```python
from build123d import *

# Parameters (mm, degrees)
SKETCH1_R               = 63.5
BOSS_EXTRUDE1_DEPTH     = 762
CUT_EXTRUDE1_DEPTH      = 1032.82015403
CUT_EXTRUDE1_DEPTH_BACK = 387.260908
SKETCH2_W               = 765.404618736
SKETCH2_H               = 508
SKETCH3_R               = 38.1
BOSS_EXTRUDE2_DEPTH     = 203.2
FILLET1_R               = 25.4


with BuildPart() as part:
    # Sketch1 → Boss-Extrude1 (new body)
    with BuildSketch(Plane.XY):
        with BuildLine():
            Line((-475.33654421, 0), (32.66345579, 0))
            Line((32.66345579, 0), (32.66345579, 508))
            ThreePointArc((32.66345579, 508), (-317.204687381, 440.127182905), (-475.33654421, 120.739091765))
            Line((-475.33654421, 120.739091765), (-475.33654421, 0))
        make_face()
        with Locations((-94.33654421, 378.291313639)):
            Circle(SKETCH1_R, mode=Mode.SUBTRACT)
    extrude(amount=BOSS_EXTRUDE1_DEPTH)

    # Sketch2 → Cut-Extrude1 (cut, two sides: drawn at the far end of the back side and taken through both)
    with BuildSketch(Plane(origin=(0, 508, 0), x_dir=(1, 0, 0), z_dir=(0, 1, 0)).offset(-CUT_EXTRUDE1_DEPTH_BACK)):
        with Locations((-173.345287356, -381)):
            Rectangle(SKETCH2_W, SKETCH2_H)
    extrude(amount=CUT_EXTRUDE1_DEPTH + CUT_EXTRUDE1_DEPTH_BACK, mode=Mode.SUBTRACT)

    # Sketch3 → Boss-Extrude2 (add)
    with BuildSketch(Plane.XY.offset(762)):
        with Locations(Location((-333.507660116, 140.616973841, 0), (0, 0, 180))):
            Circle(SKETCH3_R)
    boss_extrude2 = extrude(amount=BOSS_EXTRUDE2_DEPTH)

    # Mirror1: Boss-Extrude2 across plane
    add(boss_extrude2.mirror(Plane.XY.offset(381)))

    # Fillet1
    fillet1_edges = [part.edges().sort_by_distance(p)[0] for p in [
        (32.66345579, 508, 63.5),
        (32.66345579, 508, 698.5),
    ]]
    fillet(fillet1_edges, radius=FILLET1_R)


solid = part.part
```
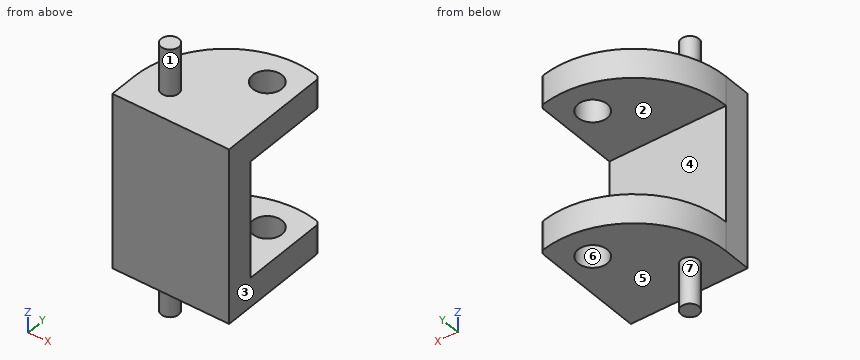
The listing builds one solid part. Answer for the finished solid, in the listing's coordinates (mm). Face numbers are marked on the shaded views. A direction names the side the tool comes from. Coordinates: 2 decimals unless noted, no trailing zeros. Loops run counter-clockwise (first coordinate to the right, second up) from the corner with the lowest first, then second, coordinate; pieces in that order, holes last. Notation, with made-up numbers: (83, -29.75) - (123, -29.75) arc R27 ccw to (123, -11.75) - close; hole circle Ø6 at (86.25, 6). An arc over 180 degrees is marked (long way). Write item = value, one per line.
1) Section B-B (x = -131) is taken. Determine the outline of the cut face in (y, z) (3 decimals).
Responses:
outline = (0, 0) - (326.445, 0) - (326.445, 127) - (120.739, 127) - (120.739, 635) - (326.445, 635) - (326.445, 762) - (0, 762) - close; (430.138, 0) - (518.244, 0) - (518.244, 127) - (430.138, 127) - close; (430.138, 635) - (518.244, 635) - (518.244, 762) - (430.138, 762) - close
2) Which of the six approach directions +Z, -Z, +X, -X, +Y, -Y give full straight-line access (tool end or side, diameter ignored) to the marked faces 1, 2 and 3?
Responses:
face_1 = +Z
face_2 = +X, -X, +Y
face_3 = +Z, -Z, +X, +Y, -Y
3) Section C-C (y = 470) is taken. Determine the outline of the cut face in (x, z).
Responses:
outline = (-271.99, 0) - (32.66, 0) - (32.66, 127) - (-271.99, 127) - close; (-271.99, 635) - (32.66, 635) - (32.66, 762) - (-271.99, 762) - close
4) Determine the mould class of the marked faces 4, 5, 6 and 7 for opening direction Y: pulls with the +Y half, pulls with the -Y half, needs draft (parallel to the pull), parting line crosses it, or undercut.
Responses:
face_4 = pulls with the +Y half
face_5 = needs draft
face_6 = undercut
face_7 = parting line crosses it
5) Section D-D (z = 552.5) is taken. Determine the outline of the cut face in (x, y).
Responses:
outline = (-475.34, 0) - (32.66, 0) - (32.66, 120.74) - (-475.34, 120.74) - close
6) Section A-A (y = 407) is taken. Determine the outline of the cut face in (x, z).
Responses:
outline = (-355.41, 0) - (-150.98, 0) - (-150.98, 127) - (-355.41, 127) - close; (-355.41, 635) - (-150.98, 635) - (-150.98, 762) - (-355.41, 762) - close; (-37.7, 0) - (32.66, 0) - (32.66, 127) - (-37.7, 127) - close; (-37.7, 635) - (32.66, 635) - (32.66, 762) - (-37.7, 762) - close
7) Find the intervals of material crossed by line 1 along Z through (x, y) = (-21, 381); line 2 along Z through (x, y) = (-320.5, 31.5); line 3 along Y through (x, z) = (-286.5, 227), in increasing order.
Responses:
line_1 = 0 to 127, 635 to 762
line_2 = 0 to 762
line_3 = 0 to 120.74
8) Each of these flat-tipped pins is pushed along its axis until it touches: P1, Ø2, axis at x = -361, z = 776, coming from the -Y side; P2, Ø5, axis at x = -164.5, y = 62.5, coming from the +Z side; P3, Ø4, axis at x = -150, z = 227.5, coming from the +Y side. Where does it stop, or does it pass through?
Responses:
P1 = 113.24
P2 = 762
P3 = 120.74
